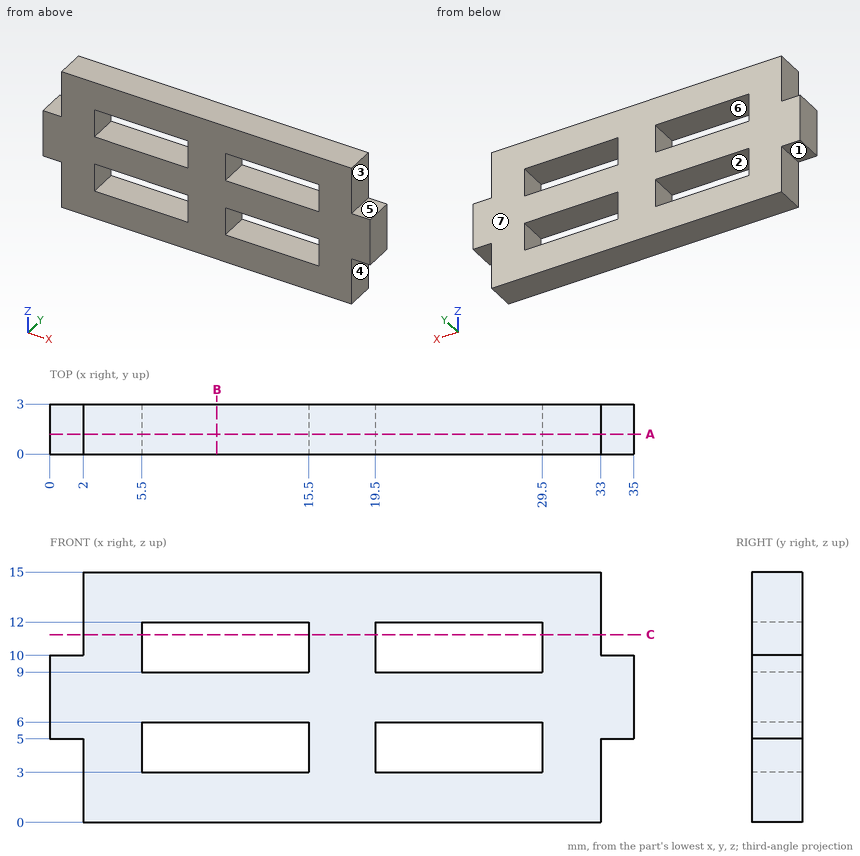
Print and shaded views of the part. All mm, measured from the part's lowest x, y and z. A direction names the side the tool comes from. Give positions to 0.01 mm unless a question says otherwise; leave off trailing zeros. Order: outer loops, then holes, each group sorted by start corner. A loop starts at its lowest first (then second) coordinate and runs counter-clockwise, first axis right, second up. Notation, with made-up numbers: (76, 76) -> (81, 76) arc R12 cw to (81, 95) -> close; hole circle Ø11 at (25.25, 54). An arc over 180 degrees is marked (long way). Use CSV: the item, a comma, the result in double quotes.
1. Drop flat-ended pins along their axis: pin 1 (1.5 mm diameter, centred on y = 1.5, z = 4, fed in from +X); pin 2 (0.9 mm diameter, centred on y = 1.5, z = 11, fed in from -X); pin 3 (0.6 mm diameter, centred on x = 34, y = 1.5, fed in from +Z). Give the stop position or say it passes through.
Outcome:
pin 1,"x = 33"
pin 2,"x = 2"
pin 3,"z = 10"
2. Mould opens along Z. For the marked faces 5, 6 and 7 say: +Z half, -Z half, draft (parallel to the pull), parting line (faces both ways), or undercut.
Outcome:
face 5,"+Z half"
face 6,"undercut"
face 7,"draft"
3. Band-saw the part on B-B, the plane x = 10. Give the cut face in (y, z).
Outcome:
outline,"(0, 0) -> (3, 0) -> (3, 3) -> (0, 3) -> close; (0, 6) -> (3, 6) -> (3, 9) -> (0, 9) -> close; (0, 12) -> (3, 12) -> (3, 15) -> (0, 15) -> close"
4. Drill centre lines: line 1 along Z through (x, y) = (9.5, 2.8); line 2 along X through (y, z) = (1, 4); line 3 along X through (y, z) = (1.25, 1). Where is each one in solid material? Low to high. Write a range as from..to.
Outcome:
line 1,"0..3, 6..9, 12..15"
line 2,"2..5.5, 15.5..19.5, 29.5..33"
line 3,"2..33"
5. Band-saw the part on A-A, the plane y = 1.2. Give the cut face in (x, z), then the cut area to 3 significant figures.
Outcome:
outline,"(0, 5) -> (2, 5) -> (2, 0) -> (33, 0) -> (33, 5) -> (35, 5) -> (35, 10) -> (33, 10) -> (33, 15) -> (2, 15) -> (2, 10) -> (0, 10) -> close; hole (5.5, 3) -> (15.5, 3) -> (15.5, 6) -> (5.5, 6) -> close; hole (5.5, 9) -> (15.5, 9) -> (15.5, 12) -> (5.5, 12) -> close; hole (19.5, 3) -> (29.5, 3) -> (29.5, 6) -> (19.5, 6) -> close; hole (19.5, 9) -> (29.5, 9) -> (29.5, 12) -> (19.5, 12) -> close"
area,"365 mm²"
6. Band-saw the part on C-C, the plane z = 11.25. Give the cut face in (x, y).
Outcome:
outline,"(2, 0) -> (5.5, 0) -> (5.5, 3) -> (2, 3) -> close; (15.5, 0) -> (19.5, 0) -> (19.5, 3) -> (15.5, 3) -> close; (29.5, 0) -> (33, 0) -> (33, 3) -> (29.5, 3) -> close"
7. 3-axis set-ups, long thin cutter, end or side, ignore diameter. For the marked faces 1, 2, 3 and 4: which of +Z, -Z, +X, -X, +Y, -Y reach the whole face in a straight line?
Outcome:
face 1,"-Z, -X, +Y, -Y"
face 2,"+Y, -Y"
face 3,"+Z, +X, +Y, -Y"
face 4,"-Z, +X, +Y, -Y"
